Model file for the job. Use its own axes, mm. A direction names the side the tool comes from. Give positions to 0.01 mm unless a question says otherwise; leave off trailing zeros. Order: outer loops, then holes, each group sorted by start corner. A loop starts at its lowest first (then second) coordinate and runs counter-clockwise, first axis right, second up. Notation, with made-up numbers: (38, 45.5) -> (96, 45.5) arc R24 cw to (96, 59.5) -> close; hole circle Ø10 at (18, 89.5). An arc over 180 degrees is marked (long way). Use CSV: the item, a comma, the result in double quotes. Start each with the question number.
1. Cut at D-D on x = 34. List the corners of the cut face in (y, z), then the cut area to 3 significant figures.
2. Wall check: line 1 (Y direction, x = 20, z = 26.5); line 2 (Y direction, x = 70, z = 281); line 3 (X direction, y = 80, z = 274.5). Give the ranges that are in metal, low to high. Write a range as from..to.
3. Cut at A-A on x = 20. List the corners of the cut face in (y, z).
4. Pull direction Y, two halves, no side cores. Call faces 4 (the flat face through (73, 100, 152)), 5 (the flat face through (40, 49, 177)), 6 (the conical face through (69.355, 19.664, 247.921)): released by +Y, released by -Y, zero draft, split by the parting line, or undercut.
5. Cut at B-B on z = 123. List the corners of the cut face in (x, y), then the cut area to 3 significant figures.
6. Cut at C-C on y = 56. List the corners of the cut face in (x, z).
7. 3-axis set-ups, long thin cutter, end or side, ignore diameter. For faces 1 (the flat face through (20, 49, 50)), 2 (the cylindrical face through (73.715, 78.067, 274.65)), 3 (the flat face through (100, 49, 148)): which of +Z, -Z, +X, -X, +Y, -Y reach the whole face in a straight line?
8. Drop flat-ended pins along their axis: pin 1 (1.5 mm diameter, centred on y = 38.5, z = 214.5, fed in from -X); pin 2 (12 mm diameter, centred on x = 20, y = 80, fed in from +Z); pin 3 (12 mm diameter, centred on x = 30, y = 68.5, fed in from +Z). Give the stop position or say it passes through.
Solid Edge part; units mm, degrees
sketch "Sketch1" plane through (0, 0, 0) normal (0, -1, 0) x (1, 0, 0)
  line L0 (100, 0) -> (100, 300)
  line L1 (100, 300) -> (40, 300)
  line L2 (40, 300) -> (40, 50)
  line L3 (40, 50) -> (0, 50)
  line L4 (0, 50) -> (0, 0)
  line L5 (0, 0) -> (100, 0)
extrude "Protrusion1" add sketch "Sketch1" against normal blind 100
hole "Bohrung_1" at (20, 20, 50) direction (0, 0, -1) diameter 10.5 end up to next start chamfer 1 start chamfer angle 45
hole "Hole1" at (20, 80, 50) direction (0, 0, -1) diameter 10.5 end up to next start chamfer 1 start chamfer angle 45
hole "Bohrung_3" at (70, 20, 300) direction (0, 0, -1) diameter 8.376 depth 50 tip angle 118
hole "Hole2" at (70, 80, 300) direction (0, 0, -1) diameter 8.376 depth 50 tip angle 118
Verdict:
1,outline,"(0, 0) -> (100, 0) -> (100, 50) -> (0, 50) -> close"
1,area,"5,000 mm^2"
2,line 1,"0..14.75, 25.25..74.75, 85.25..100"
2,line 2,"0..15.81, 24.19..75.81, 84.19..100"
2,line 3,"40..65.81, 74.19..100"
3,outline,"(0, 0) -> (14.75, 0) -> (14.75, 49) -> (13.75, 50) -> (0, 50) -> close; (25.25, 0) -> (74.75, 0) -> (74.75, 49) -> (73.75, 50) -> (26.25, 50) -> (25.25, 49) -> close; (85.25, 0) -> (100, 0) -> (100, 50) -> (86.25, 50) -> (85.25, 49) -> close"
4,face 4,"released by +Y"
4,face 5,"zero draft"
4,face 6,"undercut"
5,outline,"(40, 0) -> (100, 0) -> (100, 100) -> (40, 100) -> close"
5,area,"6,000 mm^2"
6,outline,"(0, 0) -> (100, 0) -> (100, 300) -> (40, 300) -> (40, 50) -> (0, 50) -> close"
7,face 1,"+Z, -X, +Y, -Y"
7,face 2,"+Z"
7,face 3,"+Z, -Z, +X, +Y, -Y"
8,pin 1,"x = 40"
8,pin 2,"z = 49.75"
8,pin 3,"z = 50"
